```python
from build123d import *

# Parameters (mm, degrees)
REVOLVE1_ANGLE     = 180
CHAMFER2_SIZE      = 2
SKETCH2_R          = 1.1
CUT_EXTRUDE1_DEPTH = 10


# Read off the part's stored shape, not the designer's step: Body-Delete/Keep 1
with BuildPart() as part:
    # Sketch1 → Revolve1 (revolve)
    with BuildSketch(Plane(origin=(0, 0, 0), x_dir=(1, 0, 0), z_dir=(0, 1, 0))):
        with BuildLine():
            ThreePointArc((9, 0), (6.363961031, 6.363961031), (0, 9))
            Line((0, 9), (0, 4))
            ThreePointArc((0, 4), (2.828427125, 2.828427125), (4, 0))
            ThreePointArc((4, 0), (2.828427125, -2.828427125), (0, -4))
            Line((0, -4), (0, -9))
            ThreePointArc((0, -9), (6.363961031, -6.363961031), (9, 0))
        make_face()
    revolve(axis=Axis((0, 0, -9), (0, 0, 1)), revolution_arc=REVOLVE1_ANGLE)


with BuildPart() as body_2:
    # Split1: the piece on the far side of the plane
    add(part.part)
    split(bisect_by=Plane(origin=(0, 3, 0), x_dir=(-1, 0, 0), z_dir=(0, -1, 0)), keep=Keep.BOTTOM)


with BuildPart() as part_1:
    add(part.part)

    # Split1
    split(bisect_by=Plane(origin=(0, 3, 0), x_dir=(-1, 0, 0), z_dir=(0, -1, 0)), keep=Keep.TOP)

    # Chamfer2
    # the kernel refuses this chamfer: 2, 1.766969722 mm, written as the material it takes off along each edge
    with BuildSketch(Plane(origin=(0, 3, 0), x_dir=(1, 0, 0), z_dir=(0, 0, -1))) as chamfer2_piece_1:
        with BuildLine():
            Line((2.645751311 + CHAMFER2_SIZE, 0), (3.73710994, 1.573813021))
            ThreePointArc((3.73710994, 1.573813021), (3.297092522, 0.735230497), (2.645751311, 0))
            Line((2.645751311, 0), (2.645751311 + CHAMFER2_SIZE, 0))
        make_face()
    revolve(axis=Axis((0, 3, 0), (0, -1, 0)), mode=Mode.SUBTRACT)

    # Sketch2 → Cut-Extrude1 (cut)
    with BuildSketch(Plane.XZ):
        with Locations((0, 6.5)):
            Circle(SKETCH2_R)
        with Locations((5.629165125, -3.25)):
            Circle(SKETCH2_R)
        with Locations((-5.629165125, -3.25)):
            Circle(SKETCH2_R)
    extrude(amount=-CUT_EXTRUDE1_DEPTH, mode=Mode.SUBTRACT)


solid = part_1.part
```
Build history of the part. All positions in model axes, mm. Coordinates: 2 decimals unless noted, no trailing zeros. Order: outer loops, then holes, each group sorted by start corner. A loop starts at its lowest first (then second) coordinate and runs counter-clockwise, first axis right, second up. Notation, with made-up numbers: (73.5, -26) -> (104.5, -26) arc R23 cw to (104.5, -3) -> close; hole circle Ø7 at (38.5, 15). An arc over 180 degrees is marked (long way). Answer in a Markdown table with one row per item. Add a question column.
Q1. Band-saw the part on D-D, the plane y = 1.85. List the corners of the cut face in (x, z).
Q2. Band-saw the part on A-A, the plane z = 6.5. List the corners of the cut face in (x, y).
Q3. Wall check: line 1 along Z through (x, y) = (0, 0.7); line 2 along Z through (x, y) = (0.25, 0.2); line 3 along Z through (x, y) = (5.5, 1.75). Give the ranges that are in metal, low to high. Write a range as [from, to].
Q4. Drop flat-ended pins along their axis: pin 1 (1.5 mm diameter, centred on y = 0.5, z = -4, fed in from -X); pin 2 (2 mm diameter, centred on x = -5.63, z = -3.25, fed in from +Y); pin 3 (1 mm diameter, centred on y = 2.5, z = 3, fed in from -X). Give the stop position or say it passes through.
Q5. Band-saw the part on C-C, the plane x = 0. List the corners of the cut face in (y, z).
Q6. Mould opens along Z. For faces 1 (the face through (2, 0, 4)), 2 (the face through (6.645, 1.479, -3.671)) say: +Z half, -Z half, draft (parallel to the pull), parting line (faces both ways), or undercut.
Q7. Band-saw the part on B-B, the plane x = -6.25. List the corners of the cut face in (y, z), then the cut area to 3 significant figures.
Answers follow:
| question | item | result |
|---|---|---|
| 1 | outline | circle Ø17.62 at (0, 0); hole circle Ø2.2 at (-5.63, -3.25); hole circle Ø7.96 at (0, 0); hole circle Ø2.2 at (0, 6.5); hole circle Ø2.2 at (5.63, -3.25) |
| 2 | outline | (-6.22, 0) -> (-1.1, 0) -> (-1.1, 3) -> (-5.45, 3) arc R6.22 ccw to start; (1.1, 0) -> (6.22, 0) arc R6.22 ccw to (5.45, 3) -> (1.1, 3) -> close |
| 3 | line 1 | [-8.97, -3.94], [3.94, 5.4], [7.6, 8.97] |
| 3 | line 2 | [-8.99, -3.99], [3.99, 5.43], [7.57, 8.99] |
| 3 | line 3 | [-6.91, -4.34], [-2.16, 6.91] |
| 4 | pin 1 | x = -8.38 |
| 4 | pin 2 | through |
| 4 | pin 3 | x = -8.33 |
| 5 | outline | (0, -9) arc R9 ccw to (3, -8.49) -> (3, -4.65) -> (1.43, -3.74) arc R4 cw to (0, -4) -> close; (0, 4) arc R4 cw to (1.43, 3.74) -> (3, 4.65) -> (3, 5.4) -> (0, 5.4) -> close; (0, 7.6) -> (3, 7.6) -> (3, 8.49) arc R9 ccw to (0, 9) -> close |
| 6 | face 1 | draft |
| 6 | face 2 | undercut |
| 7 | outline | (0, -6.48) arc R6.48 ccw to (3, -5.74) -> (3, -4.16) -> (0, -4.16) -> close; (0, -2.34) -> (3, -2.34) -> (3, 5.74) arc R6.48 ccw to (0, 6.48) -> close |
| 7 | area | 32.0 mm^2 |
